Autodesk Inventor part; units mm, degrees
ref_plane "CP_XY" through (0, 0, 0) normal (1, 0, 0) x (0, 0, -1)
ref_plane "CP_YZ" through (0, 0, 0) normal (0, 0, -1) x (0, 1, 0)
ref_plane "CP_ZX" through (0, 0, 0) normal (0, 1, 0) x (1, 0, 0)
sketch "Sketch_1" plane through (0, 0, 0) normal (0, 0, 1) x (1, 0, 0)
  line L0 (0, 0) -> (-6, 0)
  line L1 (-6, 0) -> (-6, 1.5705)
  line L2 (-6, 1.5705) -> (-5.5705, 2)
  line L3 (-5.5705, 2) -> (-0.75, 2)
  line L4 (-0.75, 2) -> (0, 1.25)
  line L5 (0, 1.25) -> (0, 0)
  line L6 (0, 0) -> (-6, 0)
revolve "Revolution1" add sketch "Sketch_1" angle 360 about axis through (0, 0, 0) along (1, 0, 0)
thread "Thread1"
sketch "Sketch_2" plane through (-6, 0, 0) normal (-1, 0, 0) x (0, 1, 0)
  line L0 (-1, -0.5774) -> (0, -1.1547)
  line L1 (0, -1.1547) -> (1, -0.5774)
  line L2 (1, -0.5774) -> (1, 0.5774)
  line L3 (1, 0.5774) -> (0, 1.1547)
  line L4 (0, 1.1547) -> (-1, 0.5774)
  line L5 (-1, 0.5774) -> (-1, -0.5774)
extrude "Extrusion1" cut sketch "Sketch_2" against normal blind 1.5
sketch "Sketch_3" plane through (0, 0, 0) normal (0, 0, 1) x (1, 0, 0)
  line L0 (-3.9226, 0) -> (-4.5, 0)
  line L1 (-4.5, 0) -> (-4.5, 1)
  line L2 (-4.5, 1) -> (-3.9226, 0)
  line L3 (-3.9226, 0) -> (-4.5, 0)
revolve "Revolution2" cut sketch "Sketch_3" angle 360 about axis through (-3.9226, 0, 0) along (1, 0, 0)
ref_plane "CP_XY" through (0, 0, 0) normal (1, 0, 0) x (0, 0, -1)
ref_plane "CP_YZ" through (0, 0, 0) normal (0, 0, -1) x (0, 1, 0)
ref_plane "CP_ZX" through (0, 0, 0) normal (0, 1, 0) x (1, 0, 0)
properties part number "SET-SCREW4-6"
Here's how the part is built. I have some questions about the finished solid (model axes, mm). Give positions to 0.01 mm unless a question says otherwise; leave off trailing zeros. Loops run counter-clockwise (first coordinate to the right, second up) from the corner with the lowest first, then second, coordinate; pieces in that order, holes last. Notation, with made-up numbers: M 49,15 L 72,15 A9 cw 72,32 Z; hole C 47.5,58 d2. An arc over 180 degrees is marked long. Use one line per item in the form item = value. Start each with the question number.
Q1. I need wall thicknesses on line 1 along Y through (x, z) = (-5.2, 0.05); line 2 along Z through (x, y) = (-3.3, 0.1); line 3 along X through (y, z) = (0.9, 0.45). Which ranges of each line are inside material? Lowest first, please.
Q2. If we section it at A-A (x = -5.15): Write out the boundary of the cut face in (y, z).
Q3. Thinking about a two-plate mould opening in Z: for faces 1 (the flat face through (-5, -1, 0)), 2 (the flat face through (0, 0, 0)), 3 (the cylindrical face through (-3, 0, -2)), which applies, +Z half, -Z half, draft (parallel to the pull), parting line (faces both ways), or undercut?
Q4. If we section it at B-B (x = -1.9): Write out the boundary of the cut face in (y, z).
Q5. Will these pins go through, and if not, where does the flat tip stop? pin 1 Ø1 at (x, y) = (-4, 1) entering from -Z; pin 2 Ø0.6 at (x, z) = (-5, -0.5) entering from -Y.
Taken from the geometry:
q1.line_1 = -2 to -1, 1 to 2
q1.line_2 = -2 to 2
q1.line_3 = -4.5 to 0
q2.outline = C 0,0 d4; hole M -1,-0.58 L 0,-1.15 L 1,-0.58 L 1,0.58 L 0,1.15 L -1,0.58 Z
q3.face_1 = undercut
q3.face_2 = draft
q3.face_3 = parting line
q4.outline = C 0,0 d4
q5.pin_1 = -1.94
q5.pin_2 = -1.99
